Check sheet for the drawn part. Datum: minimum x, y, z corner. Units: mm. A direction names the side the tool comes from. Round coordinates to 2 decimals unless told otherwise and drop trailing zeros. Order: outer loops, then holes, each group sorted by start corner. A loop starts at its lowest first (then second) coordinate and runs counter-clockwise, first axis right, second up.
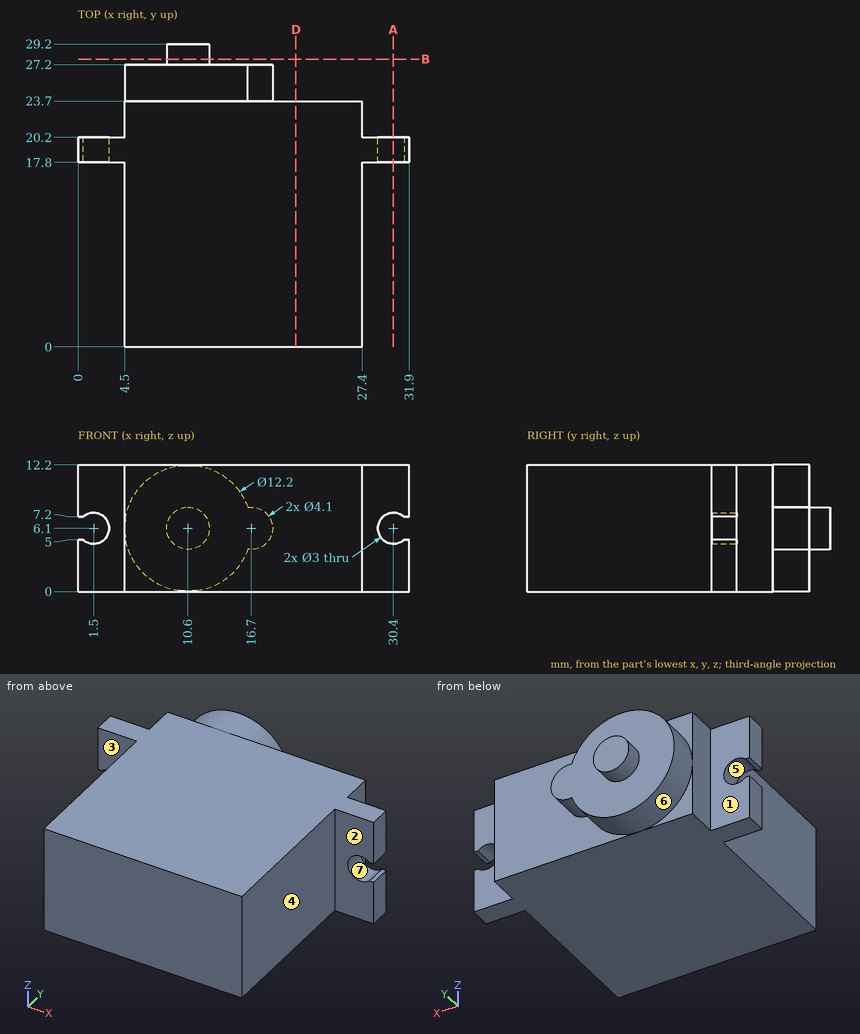
(1) Sectioned sample at A-A, the plane x = 30.4. Record the cut outline in (y, z).
Returned:
outline: (17.8, 0) - (20.2, 0) - (20.2, 4.6) - (17.8, 4.6) - close; (17.8, 7.6) - (20.2, 7.6) - (20.2, 12.2) - (17.8, 12.2) - close
(2) Material ranges on line 1 (Z direction, x = 30.4, y = 19); line 2 (X direction, y = 4.75, z = 6); line 3 (X direction, y = 18.9, z = 6.1), recorded low to high.
Returned:
line 1: z = 0 to 4.6, 7.6 to 12.2
line 2: x = 4.5 to 27.4
line 3: x = 3 to 28.9
(3) Depth check by flat-ended pin: P1, Ø2, axis at y = 11.5, z = 8, coming from the -X side; P2, Ø3, axis at x = 8, z = 10, coming from the +Y side; P3, Ø5, axis at x = 29.5, z = 4, coming from the +Y side. Enter the tip coordinate at first touch or a pass-through.
Returned:
P1: stops at x = 4.5
P2: stops at y = 27.2
P3: stops at y = 23.7
(4) Draft check along Z on the marked faces 4, 5, 6 and 7. Enter one of: released by +Z, released by -Z, zero draft, split by the parting line, or undercut.
Returned:
face 4: zero draft
face 5: undercut
face 6: split by the parting line
face 7: undercut
(5) Set-up check for the marked faces 1, 2 and 3: record each of +Z, -Z, +X, -X, +Y, -Y from which the full face is reachable in a straight line by a thin tool's end or side.
Returned:
face 1: +Z, -Z, -X, +Y
face 2: +Z, -Z, +X, -Y
face 3: +Z, -Z, -X, -Y
(6) Sectioned sample at D-D, the plane x = 21. Record the cut outline in (y, z), and give its area (3 significant figures).
Returned:
outline: (0, 0) - (23.7, 0) - (23.7, 12.2) - (0, 12.2) - close
area: 289 mm2
(7) Sectioned sample at B-B, the plane y = 27.75. Record the cut outline in (x, z).
Returned:
outline: circle Ø4.1 at (10.6, 6.1)
